The model under review builds one solid part; all positions refer to its coordinate system, in mm. Face numbers are marked on the shaded views. A direction names the side the tool comes from. Give positions to 0.01 mm unless a question says otherwise; leave off trailing zeros. Loops run counter-clockwise (first coordinate to the right, second up) from the corner with the lowest first, then second, coordinate; pieces in that order, holes last. Notation, with made-up numbers: M 18.25,28.25 L 57.25,28.25 A32 cw 57.25,65.25 Z; hole C -2,89 d3. An arc over 180 degrees is marked long. Put each result on its own line as item: value. Start each with the question number.
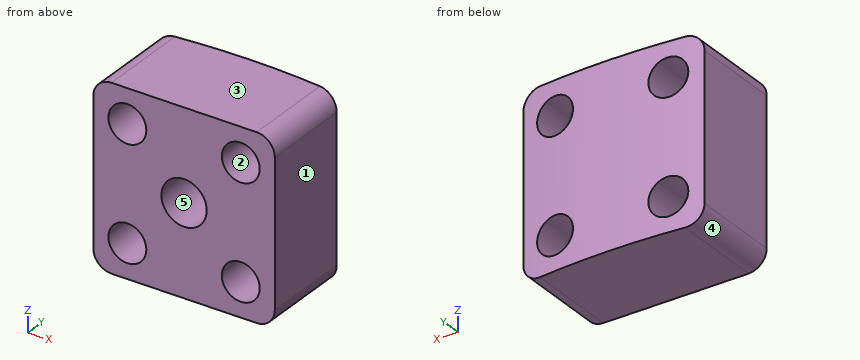
from build123d import *

# Parameters (mm, degrees)
BOSS_EXTRUDE1_DEPTH             = 12.7
BOSS_EXTRUDE1_DEPTH_BACK        = 12.7
F_1_4_0_25_DIAMETER_SLOT1_D     = 6.35
F_1_4_0_25_DIAMETER_SLOT1_DEPTH = 9.652
F_1_4_0_25_DIAMETER_SLOT1_TIP   = 1.907732465
F_4_0_209_DIAMETER_SLOT1_D      = 5.3086
F_4_0_209_DIAMETER_SLOT1_DEPTH  = 13.462
F_4_0_209_DIAMETER_SLOT1_TIP    = 1.594864341
FILLET1_R                       = 2.54


with BuildPart() as part:
    # Sketch1 → Boss-Extrude1 (new, two sides: drawn at the far end of the back side and taken through both)
    with BuildSketch(Plane.XY.offset(-BOSS_EXTRUDE1_DEPTH_BACK)):
        with BuildLine():
            Line((-12.701329683, 100.803292467), (-12.701329683, 88.103292467))
            Line((-12.701329683, 88.103292467), (12.698670317, 88.103292467))
            Line((12.698670317, 88.103292467), (12.698670317, 100.749441262))
            ThreePointArc((12.698670317, 100.749441262), (0.000359797, 101.573243718), (-12.701329683, 100.803292467))
        make_face()
    extrude(amount=BOSS_EXTRUDE1_DEPTH + BOSS_EXTRUDE1_DEPTH_BACK)

    # 1/4 (0.25) Diameter Slot1
    with Locations(Plane(origin=(0, 88.103292467, 0), x_dir=(-1, 0, 0), z_dir=(0, -1, 0))):
        with Locations((0, 0)):
            Hole(F_1_4_0_25_DIAMETER_SLOT1_D / 2, depth=F_1_4_0_25_DIAMETER_SLOT1_DEPTH)
            with Locations((0, 0, -(F_1_4_0_25_DIAMETER_SLOT1_DEPTH + F_1_4_0_25_DIAMETER_SLOT1_TIP / 2))):  # 118° drill point
                Cone(0, F_1_4_0_25_DIAMETER_SLOT1_D / 2, F_1_4_0_25_DIAMETER_SLOT1_TIP, mode=Mode.SUBTRACT)

    # #4 (0.209) Diameter Slot1
    with Locations(Plane(origin=(0, 88.103292467, 0), x_dir=(-1, 0, 0), z_dir=(0, -1, 0))):
        with Locations((-7.9375, -7.9375), (-7.9375, 7.9375), (7.9375, 7.9375), (7.9375, -7.9375)):
            Hole(F_4_0_209_DIAMETER_SLOT1_D / 2, depth=F_4_0_209_DIAMETER_SLOT1_DEPTH)
            with Locations((0, 0, -(F_4_0_209_DIAMETER_SLOT1_DEPTH + F_4_0_209_DIAMETER_SLOT1_TIP / 2))):  # 118° drill point
                Cone(0, F_4_0_209_DIAMETER_SLOT1_D / 2, F_4_0_209_DIAMETER_SLOT1_TIP, mode=Mode.SUBTRACT)

    # Fillet1
    fillet1_edges = [part.edges().sort_by_distance(p)[0] for p in [
        (-12.701329683, 94.453292467, 12.7),
        (12.698670317, 94.426366864, -12.7),
        (12.698670317, 94.426366864, 12.7),
        (-12.701329683, 94.453292467, -12.7),
    ]]
    fillet(fillet1_edges, radius=FILLET1_R)


solid = part.part
(1) To check wall thickness, follow L1, parallel to X at y = 95, z = 7.75; L2, parallel to Z at x = -8, y = 90.25; L3, parallel to X at y = 100.5, z = -5.75. State the ranges of each line that lie inside material, in increasing order. Write a range as [from, to].
(2) Insertion check: pin 1 (1 mm diameter, centred on x = -6, z = 5.5, fed in from +Y); pin 2 (8.5 mm diameter, centred on x = 0, z = 0, fed in from -Y). Each pin has a flat end and moves straight along its axis. Give the tip position at first contact, or say it passes through.
(3) We need section A-A, the plane y = 94. State how many separate pieces and enclosed holes the cut face has, plus the area to 3 significant figures.
(4) For the marked faces 4 and 5, list the 3-axis set-ups (+Z, -Z, +X, -X, +Y, -Y) from which the entire face can be reached by the end or side of a thin tool; tool diameter is ignored.
(5) Draft analysis for pull direction Z (two halves, no side actions). For the marked faces 1, 2 and 3, state which applies: +Z half, -Z half, draft (parallel to the pull), parting line (faces both ways), or undercut.
(6) We need section B-B, the plane z = -4. Write out the cut boundary in (x, y), plus the area to 3 significant figures.
Check sheet entries:
1. L1: x = [-12.7, -10.59], [-5.29, 5.29], [10.59, 12.7]
1. L2: z = [-12.7, -10.59], [-5.28, 5.28], [10.59, 12.7]
1. L3: x = [-12.7, -9.44], [-6.43, 6.43], [9.44, 12.7]
2. pin 1: stops at y = 101.44
2. pin 2: stops at y = 88.1
3. separate pieces: 1
3. enclosed holes: 5
3. area: 519 mm²
4. face 4: -Z, -X, +Y, -Y
4. face 5: -Y
5. face 1: draft
5. face 2: undercut
5. face 3: +Z half
6. outline: M -12.7,88.1 L 12.7,88.1 L 12.7,100.75 A101.6 ccw -12.7,100.8 Z
6. area: 335 mm²
